from build123d import *

# Parameters (mm, degrees)
REVOLVE1_ANGLE           = 180
REVOLVE1_OTHER_WAY_ANGLE = 90
SKETCH7_W                = 15.617438642
SKETCH7_H                = 46.497374137


with BuildPart() as part:
    # Sketch1 → Revolve1 (revolve)
    with BuildSketch(Plane(origin=(0, 0, 0), x_dir=(1, 0, 0), z_dir=(0, 1, 0))):
        with BuildLine():
            Line((-13.594162094, 76.01737396), (-13.594162094, 20))
            Line((-13.594162094, 20), (13.594162094, 20))
            Line((13.594162094, 20), (13.594162094, 76.01737396))
            ThreePointArc((13.594162094, 76.01737396), (0, 89.611536054), (-13.594162094, 76.01737396))
        make_face()
    revolve(axis=Axis((-161.278786223, 0, 0), (1, 0, 0)), revolution_arc=REVOLVE1_ANGLE)

    # Sketch1 → Revolve1 other way (revolve)
    with BuildSketch(Plane(origin=(0, 0, 0), x_dir=(1, 0, 0), z_dir=(0, 1, 0))):
        with BuildLine():
            Line((-13.594162094, 76.01737396), (-13.594162094, 20))
            Line((-13.594162094, 20), (13.594162094, 20))
            Line((13.594162094, 20), (13.594162094, 76.01737396))
            ThreePointArc((13.594162094, 76.01737396), (0, 89.611536054), (-13.594162094, 76.01737396))
        make_face()
    revolve(axis=Axis((-161.278786223, 0, 0), (-1, 0, 0)), revolution_arc=REVOLVE1_OTHER_WAY_ANGLE)

    # Sketch7 → Cut-Revolve1 (revolve, cut)
    with BuildSketch(Plane.XY):
        with Locations((-0.354941787, 81.281669295)):
            Rectangle(SKETCH7_W, SKETCH7_H)
    revolve(axis=Axis((-109.322070492, 0, 0), (1, 0, 0)), mode=Mode.SUBTRACT)


solid = part.part
Check sheet for the modelled part. Datum: model origin and axes. Units: mm. A direction names the side the tool comes from. Round coordinates to 2 decimals unless told otherwise and drop trailing zeros. Write each loop counter-clockwise with the first axis right and the second up, starting at its lowest first coordinate (ties: lowest second). Pieces come first, ordered by that corner, then holes. Notation, with made-up numbers: (35.5, 30) -> (78.5, 30) arc R20 cw to (78.5, 49) -> close; hole circle Ø6 at (-14, 75.5). An arc over 180 degrees is marked (long way). Answer as CSV lines item,"result". Start each with the question number.
1) Release check for a two-part mould opening along X. For faces 4 (the flat face through (13.594, 16, -18)), 5 (the cylindrical face through (-0.246, 39.66, -42.367)), 6 (the flat face through (0, 0, 47)) record: pulls with the +X half, pulls with the -X half, needs draft (parallel to the pull), parting line crosses it, or undercut.
2) Section check B-B on x = 11. Enter the section's corners in (y, z), and give its area (3 significant figures).
3) Go/stop test with flat-tipped pins: P1, Ø5, axis at x = -10, z = 33.5, coming from the +Y side; P2, Ø10, axis at x = -2.5, y = 43, coming from the -Z side; P3, Ø1.5, axis at x = -10.5, y = 16, coming from the -Z side. Record where each tip stops, or that it passes through.
4) Material ranges on line 1 (X direction, y = -57.5, z = -58); line 2 (X direction, y = -35.5, z = -79); line 3 (Z direction, x = 6, y = 10.5), recorded low to high. Write a range as from..to.
5) Tool access check on faces 1 (the flat face through (0, -47, 0)), 2 (the flat face through (-13.594, 16, -16)), 3 (the flat face through (-8.164, 39, -45)). Record the directions out of +Z, -Z, +X, -X, +Y, -Y that give a thin tool (end or side, any length) a straight path to the whole face; none if there is none.
6) Section check A-A on x = -2. Enter the section's corners in (y, z).
Found:
1,face 4,"pulls with the +X half"
1,face 5,"undercut"
1,face 6,"needs draft"
2,outline,"(-84, 0) arc R84 ccw (long way) to (0, 84) -> (0, 20) arc R20 cw (long way) to (-20, 0) -> close"
2,area,"15,700 mm^2"
3,P1,"stops at y = 80.86"
3,P2,"stops at z = -43.86"
3,P3,"stops at z = -83.99"
4,line 1,"x = -12.36..-8.16, 7.45..12.36"
4,line 2,"x = -8.52..-8.16, 7.45..8.52"
4,line 3,"z = -57.08..-17.02, 17.02..57.08"
5,face 1,"+Z, +X, -X, -Y"
5,face 2,"+Z, -Z, -X, +Y, -Y"
5,face 3,"none"
6,outline,"(-58.03, 0) arc R58.03 ccw (long way) to (0, 58.03) -> (0, 20) arc R20 cw (long way) to (-20, 0) -> close"
